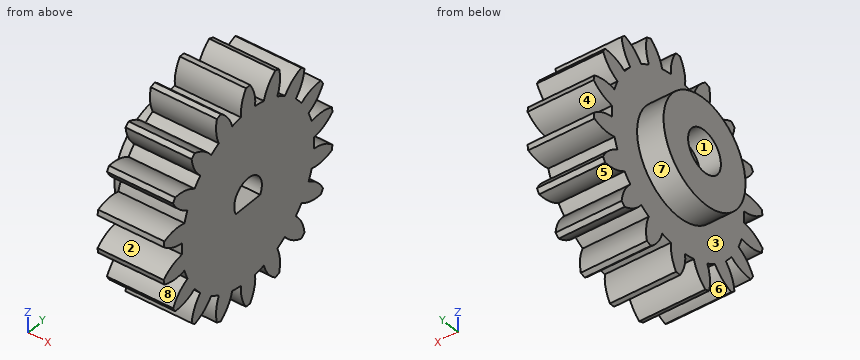
```python
from build123d import *

# Parameters (mm, degrees)
BASPROSKE_W         = 6.35
BASPROSKE_H         = 10.583333333
TOOTHCUT_DEPTH      = 17.258425166
TEETHCUTS_COUNT     = 18
TEETHCUTS_ANGLE     = 340
BORSKE_R            = 0.396875
BORE_DEPTH          = 50.8000508
CUT_EXTRUDE1_DEPTH  = 17.180937051
SKETCH2_R           = 5.08
BOSS_EXTRUDE1_DEPTH = 2.54
SKETCH3_R           = 2.032
CUT_EXTRUDE2_DEPTH  = 2.0066


with BuildPart() as part:
    # BasProSke → Base-Revolve (revolve)
    with BuildSketch(Plane(origin=(0, 0, 0), x_dir=(1, 0, 0), z_dir=(0, 1, 0)), mode=Mode.PRIVATE) as base_revolve_sk:
        with Locations((3.175, 5.291666667)):
            Rectangle(BASPROSKE_W, BASPROSKE_H)
    revolve(base_revolve_sk.sketch.rotate(Axis((-10, 0, 0), (1, 0, 0)), 180), axis=Axis((-10, 0, 0), (1, 0, 0)))

    # TooCutSke → ToothCut (cut, through all)
    with BuildSketch(Plane(origin=(0, 0, 0), x_dir=(0, 0, -1), z_dir=(1, 0, 0))):
        with BuildLine():
            ThreePointArc((0.544428341, 8.186116016), (0, 8.2042), (-0.544428341, 8.186116016))
            ThreePointArc((-0.544428341, 8.186116016), (-0.878937427, 9.427133228), (-1.607072268, 10.486302574))
            ThreePointArc((-1.607072268, 10.486302574), (0, 10.608733333), (1.607072268, 10.486302574))
            ThreePointArc((1.607072268, 10.486302574), (0.878937427, 9.427133228), (0.544428341, 8.186116016))
        make_face()
    toothcut = extrude(amount=TOOTHCUT_DEPTH, mode=Mode.SUBTRACT)

    # TeethCuts: ToothCut ×18 about axis
    teethcuts_axis = Axis((-10, 0, 0), (1, 0, 0))
    for i in range(1, TEETHCUTS_COUNT):
        add(toothcut.rotate(teethcuts_axis, i * TEETHCUTS_ANGLE / (TEETHCUTS_COUNT - 1)), mode=Mode.SUBTRACT)

    # BorSke → Bore (cut, symmetric)
    with BuildSketch(Plane(origin=(0, 0, 0), x_dir=(0, 0, -1), z_dir=(1, 0, 0))):
        with Locations(Location((0, 0, 0), (0, 0, 180))):
            Circle(BORSKE_R)
    extrude(amount=BORE_DEPTH, both=True, mode=Mode.SUBTRACT)

    # Sketch1 → Cut-Extrude1 (cut, through all)
    with BuildSketch(Plane(origin=(6.35, 0, 0), x_dir=(0, 0, -1), z_dir=(1, 0, 0))):
        with BuildLine():
            Line((0.8255, -1.502684265), (0.8255, 1.502684265))
            ThreePointArc((0.8255, 1.502684265), (-1.7145, 0), (0.8255, -1.502684265))
        make_face()
    extrude(amount=-CUT_EXTRUDE1_DEPTH, mode=Mode.SUBTRACT)

    # Sketch2 → Boss-Extrude1 (add)
    with BuildSketch(Plane.ZY):
        with Locations(Location((0, 0, 0), (0, 0, 180))):
            Circle(SKETCH2_R)
    extrude(amount=BOSS_EXTRUDE1_DEPTH)

    # Sketch3 → Cut-Extrude2 (cut)
    with BuildSketch(Plane.ZY.offset(2.54)):
        Circle(SKETCH3_R)
    extrude(amount=-CUT_EXTRUDE2_DEPTH, mode=Mode.SUBTRACT)


solid = part.part
```
Model file for the job. Use its own axes, mm. Face numbers are marked on the shaded views. A direction names the side the tool comes from. Round coordinates to 2 decimals unless told otherwise and drop trailing zeros. Write each loop counter-clockwise with the first axis right and the second up, starting at its lowest first coordinate (ties: lowest second). Pieces come first, ordered by that corner, then holes. Notation, with made-up numbers: M 22.25,27 L 71.25,27 A27 cw 71.25,57 Z; hole C 62.25,68.25 d6. An arc over 180 degrees is marked long. Put each result on its own line as item: value.
Item 1: Probe L1, parallel to Y at x = 3.75, z = 0; L2, parallel to Z at x = 2.5, y = 0; L3, parallel to Y at x = -0.95, z = 0. List the from-to ranges inside material, lowest first. Write a range as from..to.
Responses:
L1: -8.2..-1.71, 1.71..8.2
L2: -10.58..-0.83, 1.71..10.58
L3: -5.08..-2.03, 2.03..5.08
Item 2: Cut at B-B (y = 0). List the corners of the cut face in (x, z), and give its area (3 significant figures).
Responses:
outline: M -2.54,-5.08 L 0,-5.08 L 0,-10.58 L 6.35,-10.58 L 6.35,-0.83 L 0,-0.83 L 0,1.71 L 6.35,1.71 L 6.35,10.58 L 0,10.58 L 0,5.08 L -2.54,5.08 L -2.54,2.03 L -0.53,2.03 L -0.53,-2.03 L -2.54,-2.03 Z
area: 136 mm²
Item 3: Flat gauge pin, fed straight in: P1, Ø1, axis at x = 0.5, z = -4.5, coming from the -Y side. Where does the tip first touch, or does it go through?
Responses:
P1: y = -9.26
Item 4: Tool access for the marked faces 5, 6, 7 and 8: list every direction of +Z, -Z, +X, -X, +Y, -Y with a clear straight run to the whole face (end or side of a thin tool).
Responses:
face 5: +X, -X
face 6: -Z, +X, -X
face 7: -X
face 8: +X, -X, -Y
Item 5: Cut at C-C (z = 0). List the corners of the cut face in (x, y).
Responses:
outline: M -2.54,-5.08 L 0,-5.08 L 0,-8.2 L 6.35,-8.2 L 6.35,-1.71 L 0,-1.71 L 0,1.71 L 6.35,1.71 L 6.35,8.2 L 0,8.2 L 0,5.08 L -2.54,5.08 L -2.54,2.03 L -0.53,2.03 L -0.53,-2.03 L -2.54,-2.03 Z
Item 6: Cut at A-A (z = 8.75). List the corners of the cut face in (x, y), and give its area (3 significant figures).
Responses:
outline: M 0,-3.96 L 6.35,-3.96 L 6.35,-2.27 L 0,-2.27 Z; M 0,-0.89 L 6.35,-0.89 L 6.35,0.89 L 0,0.89 Z; M 0,2.27 L 6.35,2.27 L 6.35,3.96 L 0,3.96 Z
area: 32.8 mm²
Item 7: Cut at D-D (y = 6.25). List the corners of the cut face in (x, z).
Responses:
outline: M 0,-8.15 L 6.35,-8.15 L 6.35,-6.06 L 0,-6.06 Z; M 0,-5.31 L 6.35,-5.31 L 6.35,5.31 L 0,5.31 Z; M 0,6.06 L 6.35,6.06 L 6.35,8.15 L 0,8.15 Z
Item 8: Mould opens along Y. For the marked faces 1, 2, 3 and 4 say: +Y half, -Y half, draft (parallel to the pull), parting line (faces both ways), or undercut.
Responses:
face 1: undercut
face 2: -Y half
face 3: draft
face 4: +Y half
